from build123d import *

# Parameters (mm, degrees)
SKETCH1_R           = 125
SKETCH1_R_2         = 37.5
SKETCH1_R_3         = 5
BOSS_EXTRUDE2_DEPTH = 10
SKETCH2_R           = 111.468965798
SKETCH2_R_2         = 83.303584862
BOSS_EXTRUDE3_DEPTH = 10.001
SKETCH2_2_R         = 111.468965798
SKETCH2_2_R_2       = 83.303584862
BOSS_EXTRUDE4_DEPTH = 0.001


with BuildPart() as part:
    # Sketch1 → Boss-Extrude2 (new body)
    with BuildSketch(Plane.XY):
        Circle(SKETCH1_R)
        Circle(SKETCH1_R_2, mode=Mode.SUBTRACT)
        with Locations((0, 45)):
            Circle(SKETCH1_R_3, mode=Mode.SUBTRACT)
        with Locations((0, 60)):
            Circle(SKETCH1_R_3, mode=Mode.SUBTRACT)
        with Locations((0, 75)):
            Circle(SKETCH1_R_3, mode=Mode.SUBTRACT)
        with Locations((0, 90)):
            Circle(SKETCH1_R_3, mode=Mode.SUBTRACT)
        with Locations((0, 105)):
            Circle(SKETCH1_R_3, mode=Mode.SUBTRACT)
        with Locations((82.092305659, 65.466429195)):
            Circle(SKETCH1_R_3, mode=Mode.SUBTRACT)
        with Locations((70.364833422, 56.114082167)):
            Circle(SKETCH1_R_3, mode=Mode.SUBTRACT)
        with Locations((58.637361185, 46.761735139)):
            Circle(SKETCH1_R_3, mode=Mode.SUBTRACT)
        with Locations((46.909888948, 37.409388112)):
            Circle(SKETCH1_R_3, mode=Mode.SUBTRACT)
        with Locations((35.182416711, 28.057041084)):
            Circle(SKETCH1_R_3, mode=Mode.SUBTRACT)
        with Locations((102.367430779, -23.364698065)):
            Circle(SKETCH1_R_3, mode=Mode.SUBTRACT)
        with Locations((87.743512096, -20.026884056)):
            Circle(SKETCH1_R_3, mode=Mode.SUBTRACT)
        with Locations((73.119593414, -16.689070047)):
            Circle(SKETCH1_R_3, mode=Mode.SUBTRACT)
        with Locations((58.495674731, -13.351256037)):
            Circle(SKETCH1_R_3, mode=Mode.SUBTRACT)
        with Locations((43.871756048, -10.013442028)):
            Circle(SKETCH1_R_3, mode=Mode.SUBTRACT)
        with Locations((45.557792607, -94.60173113)):
            Circle(SKETCH1_R_3, mode=Mode.SUBTRACT)
        with Locations((39.049536521, -81.087198111)):
            Circle(SKETCH1_R_3, mode=Mode.SUBTRACT)
        with Locations((32.541280434, -67.572665093)):
            Circle(SKETCH1_R_3, mode=Mode.SUBTRACT)
        with Locations((26.033024347, -54.058132074)):
            Circle(SKETCH1_R_3, mode=Mode.SUBTRACT)
        with Locations((19.52476826, -40.543599056)):
            Circle(SKETCH1_R_3, mode=Mode.SUBTRACT)
        with Locations((-45.557792607, -94.60173113)):
            Circle(SKETCH1_R_3, mode=Mode.SUBTRACT)
        with Locations((-39.049536521, -81.087198111)):
            Circle(SKETCH1_R_3, mode=Mode.SUBTRACT)
        with Locations((-32.541280434, -67.572665093)):
            Circle(SKETCH1_R_3, mode=Mode.SUBTRACT)
        with Locations((-26.033024347, -54.058132074)):
            Circle(SKETCH1_R_3, mode=Mode.SUBTRACT)
        with Locations((-19.52476826, -40.543599056)):
            Circle(SKETCH1_R_3, mode=Mode.SUBTRACT)
        with Locations((-102.367430779, -23.364698065)):
            Circle(SKETCH1_R_3, mode=Mode.SUBTRACT)
        with Locations((-87.743512096, -20.026884056)):
            Circle(SKETCH1_R_3, mode=Mode.SUBTRACT)
        with Locations((-73.119593414, -16.689070047)):
            Circle(SKETCH1_R_3, mode=Mode.SUBTRACT)
        with Locations((-58.495674731, -13.351256037)):
            Circle(SKETCH1_R_3, mode=Mode.SUBTRACT)
        with Locations((-43.871756048, -10.013442028)):
            Circle(SKETCH1_R_3, mode=Mode.SUBTRACT)
        with Locations((-82.092305659, 65.466429195)):
            Circle(SKETCH1_R_3, mode=Mode.SUBTRACT)
        with Locations((-70.364833422, 56.114082167)):
            Circle(SKETCH1_R_3, mode=Mode.SUBTRACT)
        with Locations((-58.637361185, 46.761735139)):
            Circle(SKETCH1_R_3, mode=Mode.SUBTRACT)
        with Locations((-46.909888948, 37.409388112)):
            Circle(SKETCH1_R_3, mode=Mode.SUBTRACT)
        with Locations((-35.182416711, 28.057041084)):
            Circle(SKETCH1_R_3, mode=Mode.SUBTRACT)
    extrude(amount=BOSS_EXTRUDE2_DEPTH)

    # Sketch2 → Boss-Extrude3 (add)
    with BuildSketch(Plane.XY.offset(10)):
        Circle(SKETCH2_R)
        Circle(SKETCH2_R_2, mode=Mode.SUBTRACT)
    extrude(amount=-BOSS_EXTRUDE3_DEPTH)

    # Sketch2_2 → Boss-Extrude4 (add)
    with BuildSketch(Plane.XY.offset(10)):
        Circle(SKETCH2_2_R)
        Circle(SKETCH2_2_R_2, mode=Mode.SUBTRACT)
    extrude(amount=BOSS_EXTRUDE4_DEPTH)


solid = part.part
Work out the finished part from the listing and answer in its coordinate system (mm). Give positions to 0.01 mm unless a question says otherwise; leave off trailing zeros.
Q1. For a pull along X with two mould halves and no side action, classify faces 1 (the face through (54.81, -9.97, 4.93)), 2 (the face through (-124.88, 5.5, 4.93)), 3 (the face through (16, -82, 10.001)) as released by +X, released by -X, zero draft, split by the parting line, or undercut.
Answer:
face 1: undercut
face 2: split by the parting line
face 3: zero draft
Q2. Straight lines are drawn through the part: L1, parallel to Y at x = 0, z = 5.5; L2, parallel to Y at x = -22.5, z = 1.25; L3, parallel to Y at x = 39.5, z = 3.5. For each, find the intervals that lie inside material, in ascending order.
Answer:
L1: y = -125 to -37.5, 37.5 to 40, 50 to 55, 65 to 70, 80 to 125
L2: y = -122.96 to -57.6, -50.52 to -44.56, -36.53 to -30, 30 to 122.96
L3: y = -118.59 to -12.44, -7.59 to 25.54, 30.58 to 118.59
Q3. The part is cut by section A-A on z = 7.75. State how many separate pieces and enclosed holes the cut face has, and give its area (3 significant figures).
Answer:
separate pieces: 1
enclosed holes: 22
area: 43,000 mm2
Q4. Given pin 1 (9 mm diameter, centred on x = -46.91, y = 37.41, fed in from +Z); pin 2 (6 mm diameter, centred on y = -85.5, z = 7, fed in from +X); pin 3 (3 mm diameter, centred on y = 43, z = 4, fed in from +X); pin 4 (2 mm diameter, centred on y = 27, z = 8, fed in from -X), each flat-ended and moving along its own axis, determine where each tip first touches the part or whether it passes through.
Answer:
pin 1: passes through
pin 2: stops at x = 93.91
pin 3: stops at x = 117.91
pin 4: stops at x = -122.27
